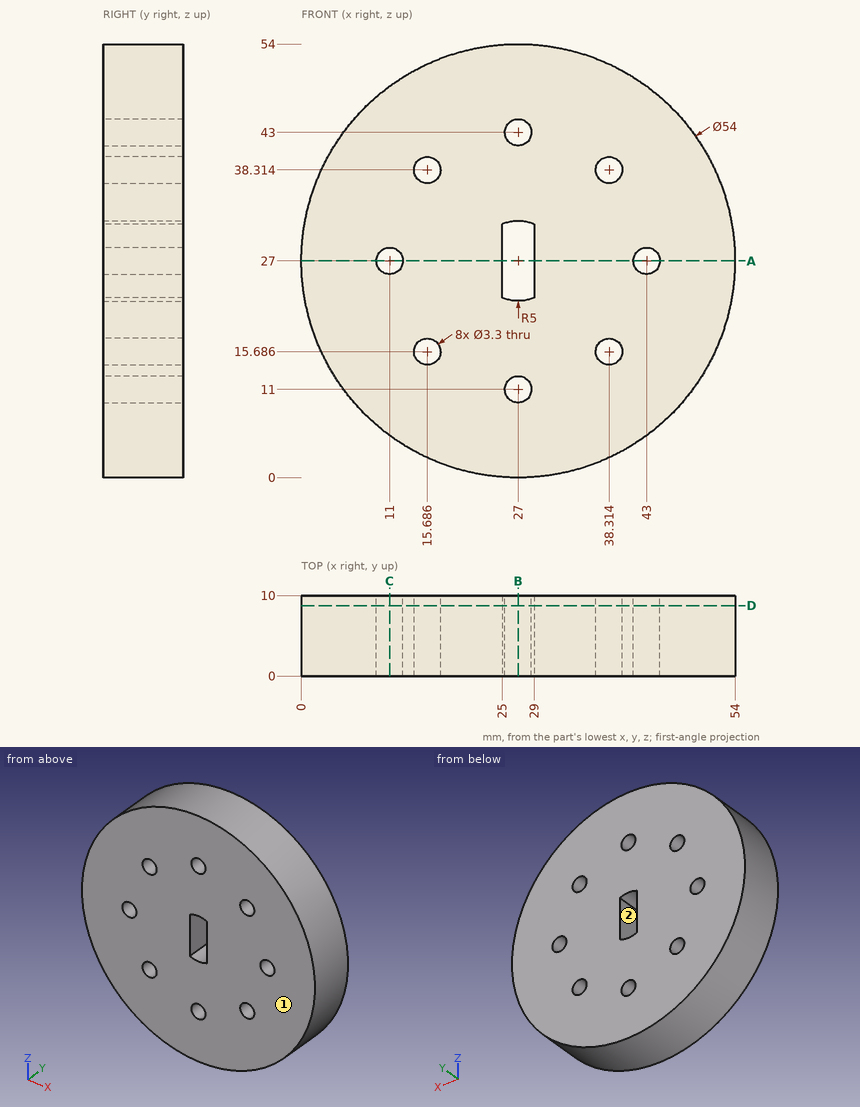
Design review of the part shown in the three views and the two pictorial views. Dimensions are in mm from the part's minimum x, y and z. A direction names the side the tool comes from. Give positions to 0.01 mm unless a question says otherwise; leave off trailing zeros. Write each loop counter-clockwise with the first axis right and the second up, starting at its lowest first coordinate (ties: lowest second). Pieces come first, ordered by that corner, then holes.
(1) Tool access review of the marked faces 1 and 2: name each direction out of +Z, -Z, +X, -X, +Y, -Y from which nothing blocks a thin tool from reaching the whole face with its end or side.
Checked values:
face 1: +Z, -Z, +X, -X, -Y
face 2: +Y, -Y
(2) Add section D-D (y = 8.75). Give the number of separate pieces and of enclosed holes in the cut face, and give its area (3 significant figures).
Checked values:
separate pieces: 1
enclosed holes: 9
area: 2,180 mm2
(3) Add section C-C (x = 11). Give the boundary of the cut face in (y, z), and give its area (3 significant figures).
Checked values:
outline: (0, 5.25) - (10, 5.25) - (10, 25.35) - (0, 25.35) - close; (0, 28.65) - (10, 28.65) - (10, 48.75) - (0, 48.75) - close
area: 402 mm2
(4) Add section A-A (z = 27). Give the boundary of the cut face in (x, y), and give its area (3 significant figures).
Checked values:
outline: (0, 0) - (9.35, 0) - (9.35, 10) - (0, 10) - close; (12.65, 0) - (25, 0) - (25, 10) - (12.65, 10) - close; (29, 0) - (41.35, 0) - (41.35, 10) - (29, 10) - close; (44.65, 0) - (54, 0) - (54, 10) - (44.65, 10) - close
area: 434 mm2
(5) Clearance check with flat-ended pins moving along their axes: pin 1 Ø4.5 at (y, z) = (2.5, 28.5) entering from -X; pin 2 Ø2 at (x, y) = (23, 6) entering from +Z; pin 3 Ø5 at (y, z) = (2, 22) entering from -X; pin 4 Ø2.5 at (x, z) = (15.69, 38.31) entering from +Y. State where each tip first meets the part, or that it passes through.
Checked values:
pin 1: stops at x = 0
pin 2: stops at z = 53.83
pin 3: stops at x = 0.12
pin 4: passes through
(6) Wall thickness on line 1 along X through (y, z) = (5.75, 27); line 2 along Z through (x, y) = (28, 4.75); line 3 along X through (y, z) = (1.5, 24): over which ranges is each line inside the solid? List them lowest first.
Checked values:
line 1: x = 0 to 9.35, 12.65 to 25, 29 to 41.35, 44.65 to 54
line 2: z = 0.02 to 9.69, 12.31 to 22.1, 31.9 to 41.69, 44.31 to 53.98
line 3: x = 0.17 to 25, 29 to 53.83
(7) Add section B-B (x = 27). Give the boundary of the cut face in (y, z).
Checked values:
outline: (0, 0) - (10, 0) - (10, 9.35) - (0, 9.35) - close; (0, 12.65) - (10, 12.65) - (10, 22) - (0, 22) - close; (0, 32) - (10, 32) - (10, 41.35) - (0, 41.35) - close; (0, 44.65) - (10, 44.65) - (10, 54) - (0, 54) - close
